Here's how the part is built. I have some questions about the finished solid (model axes, mm). A direction names the side the tool comes from. Coordinates: 2 decimals unless noted, no trailing zeros. Loops run counter-clockwise (first coordinate to the right, second up) from the corner with the lowest first, then second, coordinate; pieces in that order, holes last.
from build123d import *

# Parameters (mm, degrees)
SKETCH1_R                                     = 57.5
SKETCH1_R_2                                   = 0.5
SKETCH1_W                                     = 9.3
SKETCH1_H                                     = 9.875
BOSS_EXTRUDE1_DEPTH                           = 3
CSK_FOR_8_FLAT_HEAD_SOCKET_CAP_SCREW1_A_COUNT = 2
CSK_FOR_8_FLAT_HEAD_SOCKET_CAP_SCREW1_A_PITCH = 67.882250994
CSK_FOR_8_FLAT_HEAD_SOCKET_CAP_SCRE_2_COUNT   = 2
CSK_FOR_8_FLAT_HEAD_SOCKET_CAP_SCRE_2_PITCH   = 96
CSK_FOR_8_FLAT_HEAD_SOCKET_CAP_SCRE_3_COUNT   = 2
CSK_FOR_8_FLAT_HEAD_SOCKET_CAP_SCRE_3_PITCH   = 67.882250994
SKETCH5_W                                     = 4.0625
SKETCH5_H                                     = 9.875
CUT_EXTRUDE2_DEPTH                            = 4
SKETCH6_W                                     = 20
SKETCH6_H                                     = 25
BOSS_EXTRUDE2_DEPTH                           = 15
SKETCH7_R                                     = 4.425
CUT_EXTRUDE3_DEPTH                            = 71
SKETCH8_W                                     = 33
SKETCH8_H                                     = 3
BOSS_EXTRUDE3_DEPTH                           = 20
SKETCH9_W                                     = 33
SKETCH9_H                                     = 3
BOSS_EXTRUDE4_DEPTH                           = 20
FILLET1_R                                     = 1
FILLET2_R                                     = 5
CUT_EXTRUDE4_DEPTH                            = 4
FILLET3_R                                     = 2
SKETCH11_W                                    = 3.3
SKETCH11_H                                    = 10.3
CUT_EXTRUDE5_DEPTH                            = 3.3
SKETCH12_R                                    = 11.478689494
CUT_EXTRUDE6_DEPTH                            = 4


with BuildPart() as part:
    # Sketch1 → Boss-Extrude1 (new body)
    with BuildSketch(Plane(origin=(0, 0, 0), x_dir=(1, 0, 0), z_dir=(0, 1, 0))):
        Circle(SKETCH1_R)
        with Locations((-33.941125497, 33.941125497)):
            Circle(SKETCH1_R_2, mode=Mode.SUBTRACT)
        with Locations((33.941125497, 33.941125497)):
            Circle(SKETCH1_R_2, mode=Mode.SUBTRACT)
        with Locations((33.941125497, -33.941125497)):
            Circle(SKETCH1_R_2, mode=Mode.SUBTRACT)
        with Locations((-33.941125497, -33.941125497)):
            Circle(SKETCH1_R_2, mode=Mode.SUBTRACT)
        with Locations((1.65, 0)):
            Rectangle(SKETCH1_W, SKETCH1_H, mode=Mode.SUBTRACT)
    extrude(amount=BOSS_EXTRUDE1_DEPTH)

    # Sketch2 → CSK for #8 Flat Head Socket Cap Screw1 (revolve, cut)
    with BuildSketch(Plane(origin=(-33.941125497, 0, 33.941125497), x_dir=(0, 0, -1), z_dir=(1, 0, 0))):
        Polygon((0, 0), (0, 3), (2.45745, 3), (2.45745, 2.417901837), (4.5593, 0), align=None)
    csk_for_8_flat_head_socket_cap_screw1 = revolve(axis=Axis((-33.941125497, -6.35, 33.941125497), (0, 1, 0)), mode=Mode.SUBTRACT)

    # CSK for #8 Flat Head Socket Cap Screw1 a: CSK for #8 Flat Head Socket Cap Screw1 ×2
    with Locations(*[(i * CSK_FOR_8_FLAT_HEAD_SOCKET_CAP_SCREW1_A_PITCH, 0, 0) for i in range(1, CSK_FOR_8_FLAT_HEAD_SOCKET_CAP_SCREW1_A_COUNT)]):
        add(csk_for_8_flat_head_socket_cap_screw1, mode=Mode.SUBTRACT)

    # CSK for _8 Flat Head Socket Cap Scre 2: CSK for #8 Flat Head Socket Cap Screw1 ×2
    with Locations(*[Vector(0.707106781, 0, -0.707106781) * (i * CSK_FOR_8_FLAT_HEAD_SOCKET_CAP_SCRE_2_PITCH) for i in range(1, CSK_FOR_8_FLAT_HEAD_SOCKET_CAP_SCRE_2_COUNT)]):
        add(csk_for_8_flat_head_socket_cap_screw1, mode=Mode.SUBTRACT)

    # CSK for _8 Flat Head Socket Cap Scre 3: CSK for #8 Flat Head Socket Cap Screw1 ×2
    with Locations(*[(0, 0, -i * CSK_FOR_8_FLAT_HEAD_SOCKET_CAP_SCRE_3_PITCH) for i in range(1, CSK_FOR_8_FLAT_HEAD_SOCKET_CAP_SCRE_3_COUNT)]):
        add(csk_for_8_flat_head_socket_cap_screw1, mode=Mode.SUBTRACT)

    # Sketch5 → Cut-Extrude2 (cut, through all)
    with BuildSketch(Plane.XZ):
        with Locations((8.33125, 0)):
            Rectangle(SKETCH5_W, SKETCH5_H)
        with Locations((-5.03125, 0)):
            Rectangle(SKETCH5_W, SKETCH5_H)
    extrude(amount=-CUT_EXTRUDE2_DEPTH, mode=Mode.SUBTRACT)

    # Sketch6 → Boss-Extrude2 (add)
    with BuildSketch(Plane.XZ):
        with Locations((-30, 0)):
            Rectangle(SKETCH6_W, SKETCH6_H)
        with Locations((30, 0)):
            Rectangle(SKETCH6_W, SKETCH6_H)
    extrude(amount=BOSS_EXTRUDE2_DEPTH)

    # Sketch7 → Cut-Extrude3 (cut, through all)
    with BuildSketch(Plane.XY.offset(12.5)):
        with Locations((-32.25, -6.75)):
            Circle(SKETCH7_R)
        with Locations((32.25, -6.75)):
            Circle(SKETCH7_R)
    extrude(amount=-CUT_EXTRUDE3_DEPTH, mode=Mode.SUBTRACT)

    # Sketch8 → Boss-Extrude3 (add)
    with BuildSketch(Plane.ZY.offset(40)):
        with Locations((0, -13.5)):
            Rectangle(SKETCH8_W, SKETCH8_H)
    extrude(amount=-BOSS_EXTRUDE3_DEPTH)

    # Sketch9 → Boss-Extrude4 (add)
    with BuildSketch(Plane(origin=(40, 0, 0), x_dir=(0, 0, -1), z_dir=(1, 0, 0))):
        with Locations((0, -13.5)):
            Rectangle(SKETCH9_W, SKETCH9_H)
    extrude(amount=-BOSS_EXTRUDE4_DEPTH)

    # Fillet1
    fillet1_edges = [part.edges().sort_by_distance(p)[0] for p in [
        (-40, -13.5, -16.5),
        (-40, -13.5, 16.5),
        (-20, -13.5, -16.5),
        (-20, -13.5, 16.5),
        (40, -13.5, 16.5),
        (40, -13.5, -16.5),
        (20, -13.5, 16.5),
        (20, -13.5, -16.5),
    ]]
    fillet(fillet1_edges, radius=FILLET1_R)

    # Fillet2
    fillet2_edges = [part.edges().sort_by_distance(p)[0] for p in [
        (20, 0, 0),
        (40, 0, 0),
        (-40, 0, 0),
        (-20, 0, 0),
    ]]
    fillet(fillet2_edges, radius=FILLET2_R)

    # Sketch10 → Cut-Extrude4 (cut, through all)
    with BuildSketch(Plane.XZ):
        with BuildLine():
            Line((26.397456258, 40.686905794), (10.885548972, 16.778105482))
            ThreePointArc((10.885548972, 16.778105482), (0, 20), (-10.885548972, 16.778105482))
            Line((-10.885548972, 16.778105482), (-26.397456258, 40.686905794))
            ThreePointArc((-26.397456258, 40.686905794), (0, 48.5), (26.397456258, 40.686905794))
        make_face()
        with BuildLine():
            Line((-26.397456258, -40.686905794), (-10.885548972, -16.778105482))
            ThreePointArc((-10.885548972, -16.778105482), (0, -20), (10.885548972, -16.778105482))
            Line((10.885548972, -16.778105482), (26.397456258, -40.686905794))
            ThreePointArc((26.397456258, -40.686905794), (0, -48.5), (-26.397456258, -40.686905794))
        make_face()
    extrude(amount=-CUT_EXTRUDE4_DEPTH, mode=Mode.SUBTRACT)

    # Fillet3
    fillet3_edges = [part.edges().sort_by_distance(p)[0] for p in [
        (-26.397456258, 1.5, 40.686905794),
        (26.397456258, 1.5, 40.686905794),
        (10.885548972, 1.5, 16.778105482),
        (-10.885548972, 1.5, 16.778105482),
        (-10.885548972, 1.5, -16.778105482),
        (10.885548972, 1.5, -16.778105482),
        (26.397456258, 1.5, -40.686905794),
        (-26.397456258, 1.5, -40.686905794),
    ]]
    fillet(fillet3_edges, radius=FILLET3_R)

    # Sketch11 → Cut-Extrude5 (cut)
    with BuildSketch(Plane.XZ.offset(15)):
        with Locations((-38.35, 0)):
            Rectangle(SKETCH11_W, SKETCH11_H)
        with Locations((38.35, 0)):
            Rectangle(SKETCH11_W, SKETCH11_H)
    extrude(amount=-CUT_EXTRUDE5_DEPTH, mode=Mode.SUBTRACT)

    # Sketch12 → Cut-Extrude6 (cut, through all)
    with BuildSketch(Plane.XZ):
        Circle(SKETCH12_R)
    extrude(amount=-CUT_EXTRUDE6_DEPTH, mode=Mode.SUBTRACT)


solid = part.part
Q1. Suppose I cut it at B-B on z = 0. Write out the boundary of the cut face in (x, y) (3 decimals), and give its area (3 significant figures).
Q2. Suppose I cut it at A-A on y = -6.75. Write out the boundary of the cut face in (x, z) (3 decimals).
Q3. Will these pins go through, and if not, where does the flat tip stop? P1, Ø5, axis at y = -11, z = -6, coming from the +X side; P2, Ø8, axis at y = -8, z = 0.5, coming from the -X side; P3, Ø6, axis at x = -22.5, y = -11, coming from the +Z side.
Q4. Please list where these lines run through material, in increasing order: probe 1 along X at (y, z) = (-12.25, 11.5); probe 2 along Y at (x, z) = (-32.25, 3.75) (3 decimals); probe 3 along Y at (x, z) = (29.5, -16).
Q5. For faces 5 (the flat face through (-38, -13, -5.15)), 6 (the flat face through (20, -10, 0)), 7 (the flat face through (18.51, 1.48, -28.53)), 8 (the flat face through (-40, -10, 0)), which set-ups out of +Z, -Z, +X, -X, +Y, -Y let a thin tool reach every point of the face, with its end or its side?
Q6. Suppose I cut it at C-C on x = 0. Write out the boundary of the cut face in (y, z), and give its area (3 significant figures).
Q7. We'd pull the mould along Y, two halves only. Please class faces 1 (the flat face through (-38, -11.7, 0)), 2 (the flat face through (38, -13, 5.15)), 3 (the flat face through (30, -12, -14)), 4 (the cylindrical face through (27.83, -6.56, 0.18)): pulls with the +Y half, pulls with the -Y half, needs draft (parallel to the pull), parting line crosses it, or undercut.
Check values:
1. outline: (-57.5, 0) - (-45, 0) arc R5 cw to (-40, -5) - (-40, -11.7) - (-36.7, -11.7) - (-36.7, -15) - (-20, -15) - (-20, -5) arc R5 cw to (-15, 0) - (-11.479, 0) - (-11.479, 3) - (-57.5, 3) - close; (11.479, 0) - (15, 0) arc R5 cw to (20, -5) - (20, -15) - (36.7, -15) - (36.7, -11.7) - (40, -11.7) - (40, -5) arc R5 cw to (45, 0) - (57.5, 0) - (57.5, 3) - (11.479, 3) - close; hole circle Ø8.85 at (-32.25, -6.75); hole circle Ø8.85 at (32.25, -6.75)
1. area: 753 mm2
2. outline: (-40, -12.5) - (-36.675, -12.5) - (-36.675, 12.5) - (-40, 12.5) - close; (-27.825, -12.5) - (-20, -12.5) - (-20, 12.5) - (-27.825, 12.5) - close; (20, -12.5) - (27.825, -12.5) - (27.825, 12.5) - (20, 12.5) - close; (36.675, -12.5) - (40, -12.5) - (40, 12.5) - (36.675, 12.5) - close
3. P1: stops at x = 40
3. P2: stops at x = -40.1
3. P3: stops at z = 16.5
4. probe 1: x = -40 to -20, 20 to 40
4. probe 2: y = -15 to -11.175, -2.325 to 3
4. probe 3: y = -15 to -12, 0 to 3
5. face 5: -X, -Y
5. face 6: +Z, -Z, -Y
5. face 7: +Y, -Y
5. face 8: +Z, -Z, -X, -Y
6. outline: (0, -57.5) - (3, -57.5) - (3, -48.5) - (0, -48.5) - close; (0, -20) - (3, -20) - (3, -11.48) - (0, -11.48) - close; (0, 11.48) - (3, 11.48) - (3, 20) - (0, 20) - close; (0, 48.5) - (3, 48.5) - (3, 57.5) - (0, 57.5) - close
6. area: 105 mm2
7. face 1: pulls with the -Y half
7. face 2: needs draft
7. face 3: undercut
7. face 4: undercut
